The drawing under review shows one solid part. Ordinate dimensions are in mm from its lowest x, y, z. A direction names the side the tool comes from. Round coordinates to 2 decimals unless told otherwise and drop trailing zeros. Write each loop counter-clockwise with the first axis right and the second up, starting at its lowest first coordinate (ties: lowest second). Pieces come first, ordered by that corner, then holes. Notation, with made-up numbers: (-37, -5) -> (12, -5) arc R21 cw to (12, 12) -> close; hole circle Ø8 at (87.5, 9). An arc over 180 degrees is marked (long way). Write item = value, one per line. Start each with the question number.
Item 1: Machinability: for the marked faces 1, 2, 3 and 4, which of the approach directions +Z, -Z, +X, -X, +Y, -Y give a long, thin tool a straight path to every point of the face, cutting with its end or side? Answer none if there is none.
Item 2: Mouldability with a two-part tool opening along X and no side actions: class the marked faces 5 and 6 as released by +X, released by -X, zero draft, split by the parting line, or undercut.
Item 3: Add section D-D, the plane x = 232. State the section outline as (y, z) points, then the cut area to 3 significant figures.
Item 4: Add section B-B, the plane y = 25. State the section outline as (x, z) points, then the cut area to 3 significant figures.
Item 5: For pin 1 Ø17 at (x, z) = (29, 73) entering from +Y; pin 2 Ø14 at (x, y) = (47, 3.5) entering from -Z; pin 3 Ø4 at (y, z) = (60, 66) entering from +X, all flat-tipped, find the tip position at first contact; note any pin that passes through.
Item 6: To check wall thickness, follow L1, parallel to X at y = 3, z = 57.15; L2, parallel to Z at x = 38, y = 8; L3, parallel to X at y = 21, z = 7. State the ranges of each line that lie inside material, in increasing order.
Item 7: Add section C-C, the plane z = 104.5. State the section outline as (x, y) points, then the cut area to 3 significant figures.
Item 8: Add section A-A, the plane x = 139.7. State the section outline as (y, z) points (3 decimals), then the cut area to 3 significant figures.
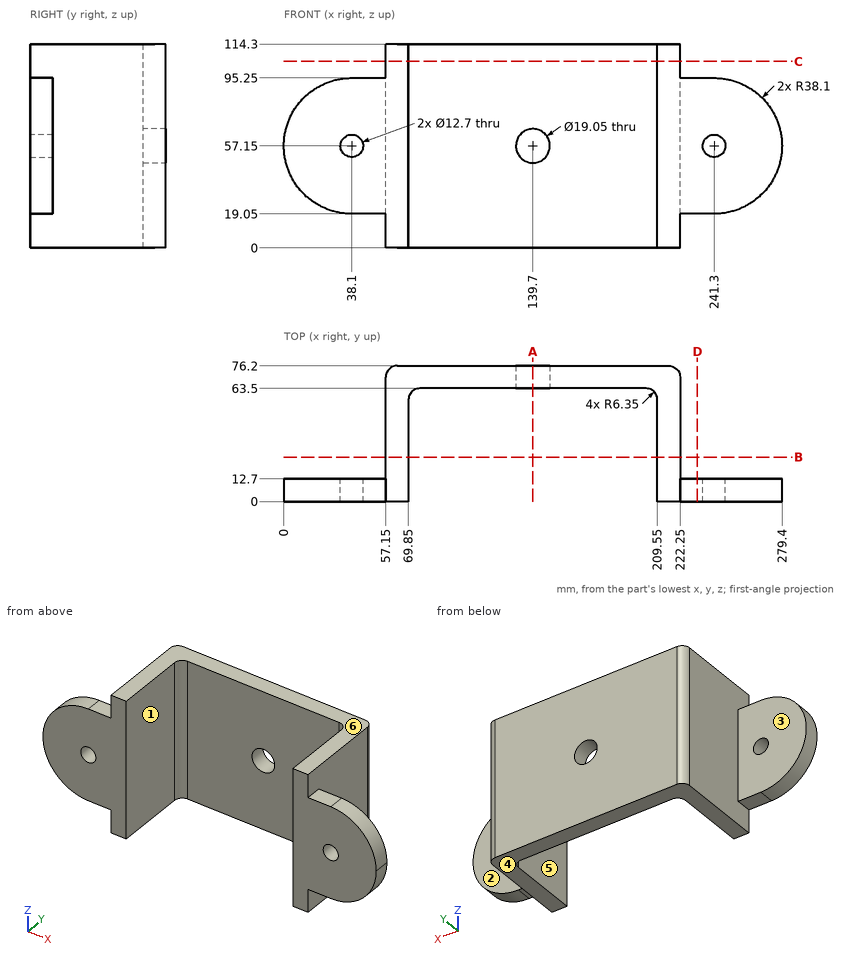
Result set:
q1.face_1 = +Z, -Z, -Y
q1.face_2 = +Z, -Z, +X, +Y
q1.face_3 = +Z, -Z, -X, +Y
q1.face_4 = -Z, +X, -X, +Y, -Y
q2.face_5 = undercut
q2.face_6 = zero draft
q3.outline = (0, 19.05) -> (12.7, 19.05) -> (12.7, 95.25) -> (0, 95.25) -> close
q3.area = 968 mm²
q4.outline = (57.15, 0) -> (69.85, 0) -> (69.85, 114.3) -> (57.15, 114.3) -> close; (209.55, 0) -> (222.25, 0) -> (222.25, 114.3) -> (209.55, 114.3) -> close
q4.area = 2,900 mm²
q5.pin_1 = 12.7
q5.pin_2 = 19.05
q5.pin_3 = 222.25
q6.L1 = 0 to 31.75, 44.45 to 69.85, 209.55 to 234.95, 247.65 to 279.4
q6.L2 = 19.05 to 50.8, 63.5 to 95.25
q6.L3 = 57.15 to 69.85, 209.55 to 222.25
q7.outline = (57.15, 0) -> (69.85, 0) -> (69.85, 57.15) arc R6.35 cw to (76.2, 63.5) -> (203.2, 63.5) arc R6.35 cw to (209.55, 57.15) -> (209.55, 0) -> (222.25, 0) -> (222.25, 69.85) arc R6.35 ccw to (215.9, 76.2) -> (63.5, 76.2) arc R6.35 ccw to (57.15, 69.85) -> close
q7.area = 3,710 mm²
q8.outline = (63.5, 0) -> (76.2, 0) -> (76.2, 47.625) -> (63.5, 47.625) -> close; (63.5, 66.675) -> (76.2, 66.675) -> (76.2, 114.3) -> (63.5, 114.3) -> close
q8.area = 1,210 mm²
